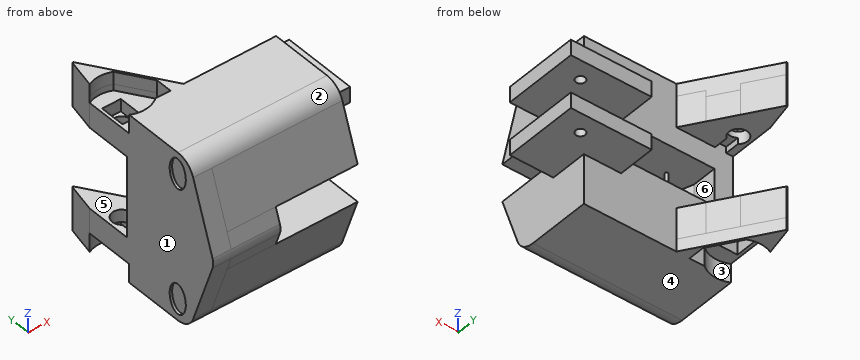
from build123d import *

# Parameters (mm, degrees)
EXTRUDE_1_DEPTH           = 30
EXTRUDE_2_DEPTH           = 210
SKETCH_8_W                = 25
SKETCH_8_H                = 120
EXTRUDE_5_DEPTH           = 70
SKETCH_9_W                = 25
SKETCH_9_H                = 60
EXTRUDE_6_DEPTH           = 60
SKETCH_10_R               = 7.5
CUT_EXTRUDE_3_DEPTH       = 402.372644808
EXTRUDE_7_DEPTH           = 60
EXTRUDE_8_REACH           = 392.16
SKETCH_12_R               = 2.5
SKETCH_14_W               = 125
SKETCH_14_H               = 50
EXTRUDE_9_DEPTH           = 120
SKETCH_15_W               = 70
SKETCH_15_H               = 70
CUT_EXTRUDE_4_DEPTH       = 10
CUT_EXTRUDE_5_DEPTH       = 20
SKETCH_17_R               = 43.471266984
CUT_EXTRUDE_6_DEPTH       = 428.317212384
EXTRUDE_10_DEPTH          = 20
EXTRUDE_11_DEPTH          = 20
CUT_EXTRUDE_7_DEPTH       = 434.012701892
CUT_EXTRUDE_8_DEPTH       = 434.012701892
EXTRUDE_19_REACH          = 446.86
EXTRUDE_20_DEPTH          = 20
EXTRUDE_21_DEPTH          = 20
EXTRUDE_START             = 20
EXTRUDE_22_DEPTH          = 20
CUT_EXTRUDE_9_DEPTH       = 30
CUT_EXTRUDE_11_DEPTH      = 407.201920232
CUT_EXTRUDE_11_DEPTH_BACK = 407.201920232
SKETCH_29_R               = 15
EXTRUDE_23_DEPTH          = 78.20324
SKETCH_33_W               = 30
SKETCH_33_H               = 40
CUT_EXTRUDE_14_DEPTH      = 20
SKETCH_34_W               = 18
SKETCH_34_H               = 35.300600551
CUT_EXTRUDE_15_DEPTH      = 10
CUT_EXTRUDE_16_DEPTH      = 10
SKETCH_36_RX              = 24.05
SKETCH_36_RY              = 15.9
SKETCH_36_R               = 15.9
CUT_EXTRUDE_17_DEPTH      = 4


with BuildPart() as part:
    # 草图1 → 凸台-拉伸1 (new body)
    with BuildSketch(Plane(origin=(0, 0, 0), x_dir=(0, 0, -1), z_dir=(1, 0, 0))):
        with BuildLine():
            Line((0, 0), (270, 0))
            Line((270, 0), (270, -100.282814983))
            ThreePointArc((270, -100.282814983), (264.178138298, -118.691056762), (248.830033233, -130.404003019))
            Line((248.830033233, -130.404003019), (142.45524498, -168.69892679))
            ThreePointArc((142.45524498, -168.69892679), (135, -170), (127.54475502, -168.69892679))
            Line((127.54475502, -168.69892679), (21.169966767, -130.404003019))
            ThreePointArc((21.169966767, -130.404003019), (5.821861702, -118.691056762), (0, -100.282814983))
            Line((0, -100.282814983), (0, 0))
        make_face()
    extrude(amount=EXTRUDE_1_DEPTH)

    # 草图2 → 凸台-拉伸2 (add)
    with BuildSketch(Plane(origin=(30, 0, 0), x_dir=(0, 0, -1), z_dir=(1, 0, 0))):
        with BuildLine():
            Line((105, -160.582814983), (105, 0))
            Line((105, 0), (0, 0))
            Line((0, 0), (0, -100.282814983))
            ThreePointArc((0, -100.282814983), (5.821861702, -118.691056762), (21.169966767, -130.404003019))
            Line((21.169966767, -130.404003019), (105, -160.582814983))
        make_face()
        with BuildLine():
            Line((270, 0), (165, 0))
            Line((165, 0), (165, -160.582814983))
            Line((165, -160.582814983), (248.830033233, -130.404003019))
            ThreePointArc((248.830033233, -130.404003019), (264.178138298, -118.691056762), (270, -100.282814983))
            Line((270, -100.282814983), (270, 0))
        make_face()
    extrude(amount=EXTRUDE_2_DEPTH)

    # 草图8 → 凸台-拉伸5 (add)
    with BuildSketch(Plane(origin=(240, 0, 0), x_dir=(0, 0, -1), z_dir=(1, 0, 0))):
        with Locations((92.5, 0)):
            Rectangle(SKETCH_8_W, SKETCH_8_H)
        with Locations((177.5, 0)):
            Rectangle(SKETCH_8_W, SKETCH_8_H)
    extrude(amount=EXTRUDE_5_DEPTH)

    # 草图9 → 凸台-拉伸6 (add)
    with BuildSketch(Plane.ZY.offset(-240)):
        with Locations((-92.5, 30)):
            Rectangle(SKETCH_9_W, SKETCH_9_H)
        with Locations((-177.5, 30)):
            Rectangle(SKETCH_9_W, SKETCH_9_H)
    extrude(amount=EXTRUDE_6_DEPTH)

    # 草图10 → 切除-拉伸3 (cut, through all)
    with BuildSketch(Plane.XY.offset(-80)):
        with Locations((270, 30)):
            Circle(SKETCH_10_R)
    extrude(amount=-CUT_EXTRUDE_3_DEPTH, mode=Mode.SUBTRACT)

    # 草图11 → 凸台-拉伸7 (add)
    with BuildSketch(Plane(origin=(0, 0, -105), x_dir=(-1, 0, 0), z_dir=(0, 0, -1))):
        with BuildLine():
            Line((-30, -40), (-30, -160.582814983))
            Line((-30, -160.582814983), (-108.203242822, -160.582814983))
            ThreePointArc((-108.203242822, -160.582814983), (-60.24964282, -106.032303748), (-30, -40))
        make_face()
    extrude(amount=EXTRUDE_7_DEPTH)

    # 草图12 → 凸台-拉伸8 (add, up to next)
    with BuildSketch(Plane.XY.offset(-165), mode=Mode.PRIVATE) as extrude_8_sk1:
        with Locations(Location((70, -45, 0), (0, 0, 180))):
            Circle(SKETCH_12_R)
    extrude_8_tool1 = extrude(extrude_8_sk1.sketch, amount=EXTRUDE_8_REACH, mode=Mode.PRIVATE) - part.part
    add(extrude_8_tool1.solids().sort_by_distance((70, -45, -165))[0])

    # 草图14 → 凸台-拉伸9 (add)
    with BuildSketch(Plane(origin=(0, 0, 0), x_dir=(1, 0, 0), z_dir=(0, 1, 0))):
        with Locations((62.5, 225)):
            Rectangle(SKETCH_14_W, SKETCH_14_H)
        with Locations((62.5, 45)):
            Rectangle(SKETCH_14_W, SKETCH_14_H)
    extrude(amount=EXTRUDE_9_DEPTH)

    # 草图15 → 切除-拉伸4 (cut)
    with BuildSketch(Plane.XY.offset(-20)):
        with Locations((35, 35)):
            Rectangle(SKETCH_15_W, SKETCH_15_H)
    extrude(amount=-CUT_EXTRUDE_4_DEPTH, mode=Mode.SUBTRACT)

    # 草图16 → 切除-拉伸5 (cut)
    with BuildSketch(Plane.XY.offset(-30)):
        Polygon((35, 15), (5, 15), (5, 55), (35, 55), (35, 35), align=None)
    extrude(amount=-CUT_EXTRUDE_5_DEPTH, mode=Mode.SUBTRACT)

    # 草图17 → 切除-拉伸6 (cut, through all)
    with BuildSketch(Plane.XY.offset(-30)):
        with Locations((19.5, 34.5)):
            Circle(SKETCH_17_R)
    extrude(amount=CUT_EXTRUDE_6_DEPTH, mode=Mode.SUBTRACT)

    # 草图18 → 凸台-拉伸10 (add)
    with BuildSketch(Plane.XY.offset(-20)):
        Polygon((11.819921283, 120), (91.211474189, 0), (87.317867735, 0), (10.741661946, 115.744614613), align=None)
    extrude(amount=EXTRUDE_10_DEPTH)

    # 草图19 → 凸台-拉伸11 (add)
    with BuildSketch(Plane.XY.offset(-20)):
        with BuildLine():
            Line((1.857343832, 74.230186717), (10.856035233, 115.571739869))
            Line((10.856035233, 115.571739869), (10.741661946, 115.744614613))
            Line((10.741661946, 115.744614613), (11.819921283, 120))
            Line((11.819921283, 120), (10.153664863, 120))
            Line((10.153664863, 120), (0, 73.352297914))
            ThreePointArc((0, 73.352297914), (0.923485284, 73.80221564), (1.857343832, 74.230186717))
        make_face()
    extrude(amount=EXTRUDE_11_DEPTH)

    # 草图20 → 切除-拉伸7 (cut, through all)
    with BuildSketch(Plane.XY.offset(-20)):
        Polygon((0, 120), (0, 73.352297914), (10.153664863, 120), align=None)
    extrude(amount=-CUT_EXTRUDE_7_DEPTH, mode=Mode.SUBTRACT)

    # 草图22 → 切除-拉伸8 (cut, through all)
    with BuildSketch(Plane.XY.offset(-20)):
        Polygon((44.899734993, 70), (70, 32.061054476), (91.211474189, 0), (125, 0), (125, 120), (11.819921283, 120), align=None)
    extrude(amount=-CUT_EXTRUDE_8_DEPTH, mode=Mode.SUBTRACT)

    # 草图23 → 凸台-拉伸19 (add, up to next)
    with BuildSketch(Plane.XY, mode=Mode.PRIVATE) as extrude_19_sk1:
        with BuildLine():
            Line((87.317867735, 0), (91.211474189, 0))
            Line((91.211474189, 0), (11.819921283, 120))
            Line((11.819921283, 120), (10.153664863, 120))
            Line((10.153664863, 120), (0, 73.352297914))
            ThreePointArc((0, 73.352297914), (0.923485284, 73.80221564), (1.857343832, 74.230186717))
            Line((1.857343832, 74.230186717), (10.856035233, 115.571739869))
            Line((10.856035233, 115.571739869), (87.317867735, 0))
        make_face()
    extrude_19_tool1 = extrude(extrude_19_sk1.sketch, amount=-EXTRUDE_19_REACH, mode=Mode.PRIVATE) - part.part
    add(extrude_19_tool1.solids().sort_by_distance((89.264671, 1.5073, 0))[0])

    # 草图24 → 凸台-拉伸20 (add)
    with BuildSketch(Plane.XY.offset(-20)):
        Polygon((87.317867735, 0), (70, 26.175884614), (70, 0), align=None)
    extrude(amount=EXTRUDE_20_DEPTH)

    # 草图25 → 凸台-拉伸21 (add)
    with BuildSketch(Plane.XY.offset(-20)):
        with BuildLine():
            Line((38.684579851, 73.509011127), (10.856035233, 115.571739869))
            Line((10.856035233, 115.571739869), (1.857343832, 74.230186717))
            ThreePointArc((1.857343832, 74.230186717), (20.351120273, 77.962934179), (38.684579851, 73.509011127))
        make_face()
    extrude(amount=EXTRUDE_21_DEPTH)

    # 草图26 → 凸台-拉伸22 (add)
    with BuildSketch(Plane(origin=(0, 0, -250), x_dir=(-1, 0, 0), z_dir=(0, 0, -1)).offset(EXTRUDE_START)):
        with BuildLine():
            Line((-70, 26.175884614), (-38.684579851, 73.509011127))
            ThreePointArc((-38.684579851, 73.509011127), (-19.323897117, 77.970910285), (0, 73.352297914))
            Line((0, 73.352297914), (-10.153664863, 120))
            Line((-10.153664863, 120), (-11.819921283, 120))
            Line((-11.819921283, 120), (-91.211474189, 0))
            Line((-91.211474189, 0), (-240, 0))
            Line((-240, 0), (-240, -100.282814983))
            Line((-240, -100.282814983), (0, -100.282814983))
            Line((0, -100.282814983), (0, -4.352297914))
            ThreePointArc((0, -4.352297914), (-23.599339693, -8.77755154), (-45.948082222, 0))
            Line((-45.948082222, 0), (-70, 0))
            Line((-70, 0), (-70, 26.175884614))
        make_face()
    extrude(amount=-EXTRUDE_22_DEPTH)

    # 草图27 → 切除-拉伸9 (cut)
    with BuildSketch(Plane(origin=(0, 0, -270), x_dir=(-1, 0, 0), z_dir=(0, 0, -1))):
        with BuildLine():
            Line((-38.684579851, 73.509011127), (-70, 26.175884614))
            Line((-70, 26.175884614), (-70, 0))
            Line((-70, 0), (-45.948082222, 0))
            ThreePointArc((-45.948082222, 0), (-23.599339693, -8.77755154), (0, -4.352297914))
            Line((0, -4.352297914), (0, 73.352297914))
            ThreePointArc((0, 73.352297914), (-19.323897117, 77.970910285), (-38.684579851, 73.509011127))
        make_face()
    extrude(amount=-CUT_EXTRUDE_9_DEPTH, mode=Mode.SUBTRACT)

    # 草图29 → 切除-拉伸11 (cut, two sides: drawn at the far end of the back side and taken through both)
    with BuildSketch(Plane(origin=(0, 0, -70), x_dir=(-1, 0, 0), z_dir=(0, 0, -1)).offset(-CUT_EXTRUDE_11_DEPTH_BACK)):
        with Locations((-20, 35)):
            Circle(SKETCH_29_R)
    extrude(amount=CUT_EXTRUDE_11_DEPTH + CUT_EXTRUDE_11_DEPTH_BACK, mode=Mode.SUBTRACT)

    # 草图30 → 凸台-拉伸23 (add)
    with BuildSketch(Plane(origin=(30, 0, 0), x_dir=(0, 0, -1), z_dir=(1, 0, 0))):
        with BuildLine():
            Line((142.45524498, -168.69892679), (165, -160.582814983))
            Line((165, -160.582814983), (105, -160.582814983))
            Line((105, -160.582814983), (127.54475502, -168.69892679))
            ThreePointArc((127.54475502, -168.69892679), (135, -170), (142.45524498, -168.69892679))
        make_face()
    extrude(amount=EXTRUDE_23_DEPTH)

    # 草图33 → 切除-拉伸14 (cut)
    with BuildSketch(Plane(origin=(0, 0, -240), x_dir=(-1, 0, 0), z_dir=(0, 0, -1))):
        with Locations((-20, 35)):
            Rectangle(SKETCH_33_W, SKETCH_33_H)
    extrude(amount=-CUT_EXTRUDE_14_DEPTH, mode=Mode.SUBTRACT)

    # 草图34 → 切除-拉伸15 (cut)
    with BuildSketch(Plane.XY.offset(-200)):
        with Locations((20, 17.650300276)):
            Rectangle(SKETCH_34_W, SKETCH_34_H)
    extrude(amount=-CUT_EXTRUDE_15_DEPTH, mode=Mode.SUBTRACT)

    # 草图35 → 切除-拉伸16 (cut)
    with BuildSketch(Plane(origin=(0, 0, -70), x_dir=(-1, 0, 0), z_dir=(0, 0, -1))):
        with BuildLine():
            Line((-11, 0), (-11, 23))
            ThreePointArc((-11, 23), (-20, 20), (-29, 23))
            Line((-29, 23), (-29, 0))
            Line((-29, 0), (-11, 0))
        make_face()
    extrude(amount=-CUT_EXTRUDE_16_DEPTH, mode=Mode.SUBTRACT)

    # 草图36 → 切除-拉伸17 (cut)
    # profile 1 of 6: a face of its own
    with BuildSketch(Plane.ZY):
        with Locations((-235.69166945, -100.008005659)):
            Ellipse(SKETCH_36_RX, SKETCH_36_RY)
        with Locations((-235.69166945, -100.008005659)):
            Circle(SKETCH_36_R, mode=Mode.SUBTRACT)
    # profile 2 of 6: a face of its own
    with BuildSketch(Plane.ZY):
        with Locations((-235.69166945, -100.008005659)):
            Ellipse(SKETCH_36_RX, SKETCH_36_RY)
        with Locations((-235.69166945, -100.008005659)):
            Circle(SKETCH_36_R, mode=Mode.SUBTRACT)
    # profile 3 of 6: a face of its own
    with BuildSketch(Plane.ZY):
        with Locations((-235.69166945, -100.008005659)):
            Circle(SKETCH_36_R)
    # profile 4 of 6: a face of its own
    with BuildSketch(Plane.ZY):
        with Locations(Location((-34.30833055, -100.008005659), (0, 0, 180))):
            Ellipse(SKETCH_36_RX, SKETCH_36_RY)
        with Locations((-34.30833055, -100.008005659)):
            Circle(SKETCH_36_R, mode=Mode.SUBTRACT)
    # profile 5 of 6: a face of its own
    with BuildSketch(Plane.ZY):
        with Locations(Location((-34.30833055, -100.008005659), (0, 0, 180))):
            Ellipse(SKETCH_36_RX, SKETCH_36_RY)
        with Locations((-34.30833055, -100.008005659)):
            Circle(SKETCH_36_R, mode=Mode.SUBTRACT)
    # profile 6 of 6: a face of its own
    with BuildSketch(Plane.ZY):
        with Locations((-34.30833055, -100.008005659)):
            Circle(SKETCH_36_R)
    extrude(amount=-CUT_EXTRUDE_17_DEPTH, mode=Mode.SUBTRACT)


solid = part.part
Geometry check sheet. Reference: the model listing, model coordinates, mm. Face numbers are marked on the shaded views. A direction names the side the tool comes from. Round coordinates to 2 decimals unless told otherwise and drop trailing zeros. Order: outer loops, then holes, each group sorted by start corner. A loop starts at its lowest first (then second) coordinate and runs counter-clockwise, first axis right, second up. Notation, with made-up numbers: M -39,23 L -24,23 A23 ccw -24,54 Z; hole C -6.75,72.25 d4. An arc over 180 degrees is marked long. Answer in a Markdown table with one row per item. Add a question column.
Item 1: Set-up check for the marked faces 4, 5 and 6: record each of +Z, -Z, +X, -X, +Y, -Y from which the full face is reachable in a straight line by a thin tool's end or side.
Item 2: Depth check by flat-ended pin: pin 1 Ø12 at (x, z) = (61.5, -261.5) entering from +Y; pin 2 Ø12 at (y, z) = (-23, -144) entering from +X; pin 3 Ø16 at (x, y) = (13.5, 44) entering from -Z; pin 4 Ø12 at (x, z) = (260, -196.5) entering from +Y. Enter the tip coordinate at first touch or a pass-through.
Item 3: Sectioned sample at C-C, the plane z = -172.5. Enter the section's corners in (x, y), plus the area to 3 significant figures.
Item 4: Sectioned sample at D-D, the plane y = -22. Enter the section's corners in (x, z).
Item 5: Material ranges on L1, parallel to Y at x = 270, z = -98; L2, parallel to Z at x = 249, y = 0.5; L3, parallel to Z at x = 89, y = -20, recorded low to high. Write a range as [from, to].
Item 6: Sectioned sample at B-B, the plane x = 212.5. Enter the section's corners in (y, z), plus the area to 3 significant figures.
Item 7: Draft check along X on the marked faces 1, 2 and 3. Enter one of: released by +X, released by -X, zero draft, split by the parting line, or undercut.
Item 8: Sectioned sample at A-A, the plane x = 270. Enter the section's corners in (y, z).
Filled in:
| question | item | result |
|---|---|---|
| 1 | face 4 | -Z, +X, -X, +Y, -Y |
| 1 | face 5 | +X, -X, +Y |
| 1 | face 6 | +X, +Y |
| 2 | pin 1 | stops at y = 53.98 |
| 2 | pin 2 | stops at x = 30 |
| 2 | pin 3 | stops at z = -220 |
| 2 | pin 4 | passes through |
| 3 | outline | M 0,-157.88 L 240,-157.88 L 240,-60 L 310,-60 L 310,60 L 180,60 L 180,0 L 0,0 Z; hole C 270,30 d15 |
| 3 | area | 49,700 mm² |
| 4 | outline | M 0,-270 L 240,-270 L 240,-190 L 310,-190 L 310,-165 L 30,-165 L 30,-105 L 310,-105 L 310,-80 L 240,-80 L 240,0 L 0,0 Z |
| 5 | L1 | y = [-60, 22.5], [37.5, 60] |
| 5 | L2 | z = [-190, -165], [-105, -80] |
| 5 | L3 | z = [-270, -165], [-105, 0] |
| 6 | outline | M -160.58,-165 L -130.4,-248.83 A32.01 ccw -100.28,-270 L 0,-270 L 0,-190 L 60,-190 L 60,-165 Z; M -160.58,-105 L 60,-105 L 60,-80 L 0,-80 L 0,0 L -100.28,0 A32.01 ccw -130.4,-21.17 Z |
| 6 | area | 32,600 mm² |
| 7 | face 1 | released by -X |
| 7 | face 2 | zero draft |
| 7 | face 3 | undercut |
| 8 | outline | M -60,-190 L 22.5,-190 L 22.5,-165 L -60,-165 Z; M -60,-105 L 22.5,-105 L 22.5,-80 L -60,-80 Z; M 37.5,-190 L 60,-190 L 60,-165 L 37.5,-165 Z; M 37.5,-105 L 60,-105 L 60,-80 L 37.5,-80 Z |
